Input: part model. Units: mm. Frame: model coordinates. Round coordinates to 2 decimals unless told otherwise and drop trailing zeros. Order: outer loops, then holes, each group sorted by start corner. A loop starts at its lowest first (then second) coordinate and runs counter-clockwise, first axis right, second up.
Item 1: Line query: L1, parallel to Y at x = 6.75, z = 0.6; L2, parallel to X at y = 1, z = 0.4; L3, parallel to Y at x = 7.5, z = 1.55. Output: solid intervals per line, ascending.
Item 2: Cut plane A-A on z = 2.05. Output: boundary loops of the cut face in (x, y), then the cut area to 3 significant figures.
Item 3: Cut plane C-C on y = -2.75. Output: boundary loops of the cut face in (x, z), then the cut area to 3 significant figures.
Item 4: First-contact query: pin 1 (5 mm diameter, centred on x = 7.78, y = -0.22, fed in from -Z); pin 2 (3 mm diameter, centred on x = -0.22, y = 7.78, fed in from +Z); pin 3 (2 mm diameter, centred on y = 8.5, z = 2.5, fed in from +X); pin 4 (3 mm diameter, centred on x = -4, z = 3.5, fed in from +Y). Flat tips, straight axial feed; report the tip coordinate or a pass-through.
Item 5: Mould query, pull axis Y, two halves, no side actions, for faces 1 (the flat face through (7, 2, 0)), 2 (the flat face through (2.09, 2.15, 1.48)), 3 (the flat face through (-1.83, 10.9, 2.96)). Classes: released by +Y, released by -Y, zero draft, split by the parting line, or undercut.
Item 6: Cut plane D-D on z = 3.5. Output: boundary loops of the cut face in (x, y).
Item 7: Cut plane B-B on x = 11.75. Output: boundary loops of the cut face in (y, z), then the cut area to 3 significant figures.
```python
from build123d import *

# Parameters (mm, degrees)
EXTRUDE_1_DEPTH     = 13
EXTRUDE_2_DEPTH     = 3
SKETCH_4_R          = 1.6
CUT_EXTRUDE_1_DEPTH = 10


with BuildPart() as part:
    # 草图3 → 凸台-拉伸1 (new body)
    with BuildSketch(Plane(origin=(0, 0, 0), x_dir=(0, 0, -1), z_dir=(0.7071067811865488, 0.7071067811865464, 0))):
        with BuildLine():
            Line((0, 3), (0, 9))
            Line((0, 9), (-6, 9))
            Line((-6, 9), (-6, -9))
            Line((-6, -9), (0, -9))
            Line((0, -9), (0, -3))
            ThreePointArc((0, -3), (-3, 0), (0, 3))
        make_face()
    extrude(amount=EXTRUDE_1_DEPTH)

    # 草图5 → 凸台-拉伸2 (add)
    with BuildSketch(Plane(origin=(0, 0, 0), x_dir=(0, 0, 1), z_dir=(-0.7071067811865488, -0.7071067811865462, 0))):
        with BuildLine():
            Line((0, -1), (0, -3))
            ThreePointArc((0, -3), (2.121320344, -2.121320344), (3, 0))
            ThreePointArc((3, 0), (2.121320344, 2.121320344), (0, 3))
            Line((0, 3), (0, 1))
            ThreePointArc((0, 1), (0.707106781, 0.707106781), (1, 0))
            ThreePointArc((1, 0), (0.707106781, -0.707106781), (0, -1))
        make_face()
    extrude(amount=-EXTRUDE_2_DEPTH)

    # 草图4 → 切除-拉伸1 (cut)
    with BuildSketch(Plane.XY.offset(6)):
        with Locations((-0.224049788, 7.775950212)):
            Circle(SKETCH_4_R)
        with Locations((7.775950212, -0.224049788)):
            Circle(SKETCH_4_R)
    extrude(amount=-CUT_EXTRUDE_1_DEPTH, mode=Mode.SUBTRACT)


solid = part.part
```
From the geometry:
1. L1: y = -5.98 to -1.45, 1 to 2.59, 10.91 to 11.63
1. L2: x = -1 to -0.3, 2.3 to 3.24, 5.2 to 6.75, 8.81 to 13.73
1. L3: y = -5.23 to -1.8, 1.35 to 3.87
2. outline: (-6.36, 6.36) - (6.36, -6.36) - (15.56, 2.83) - (10.74, 7.64) - (3.67, 0.57) - (0.57, 3.67) - (7.64, 10.74) - (2.83, 15.56) - close; hole circle Ø3.2 at (-0.22, 7.78); hole circle Ø3.2 at (7.78, -0.22)
2. area: 174 mm2
3. outline: (2.75, 0) - (9.98, 0) - (9.98, 6) - (2.75, 6) - close
3. area: 43.4 mm2
4. pin 1: stops at z = 0
4. pin 2: passes through
4. pin 3: stops at x = 10.88
4. pin 4: stops at y = 10.23
5. face 1: zero draft
5. face 2: undercut
5. face 3: released by +Y
6. outline: (-6.36, 6.36) - (6.36, -6.36) - (15.56, 2.83) - (2.83, 15.56) - close; hole circle Ø3.2 at (-0.22, 7.78); hole circle Ø3.2 at (7.78, -0.22)
7. outline: (-0.98, 0) - (6.63, 0) - (6.63, 6) - (-0.98, 6) - close
7. area: 45.7 mm2
